Job drawing, mm, ordinate dimensions from the low corner. One solid piece. Round coordinates to 2 decimals unless told otherwise and drop trailing zeros. Order: outer loops, then holes, each group sorted by start corner. A loop starts at its lowest first (then second) coordinate and runs counter-clockwise, first axis right, second up. Notation, with made-up numbers: (-30, 5) -> (12, 5) arc R21 cw to (12, 27) -> close; hole circle Ø6 at (87, 13). An arc over 180 degrees is marked (long way). Use CSV: the item, a comma, the result in double quotes.
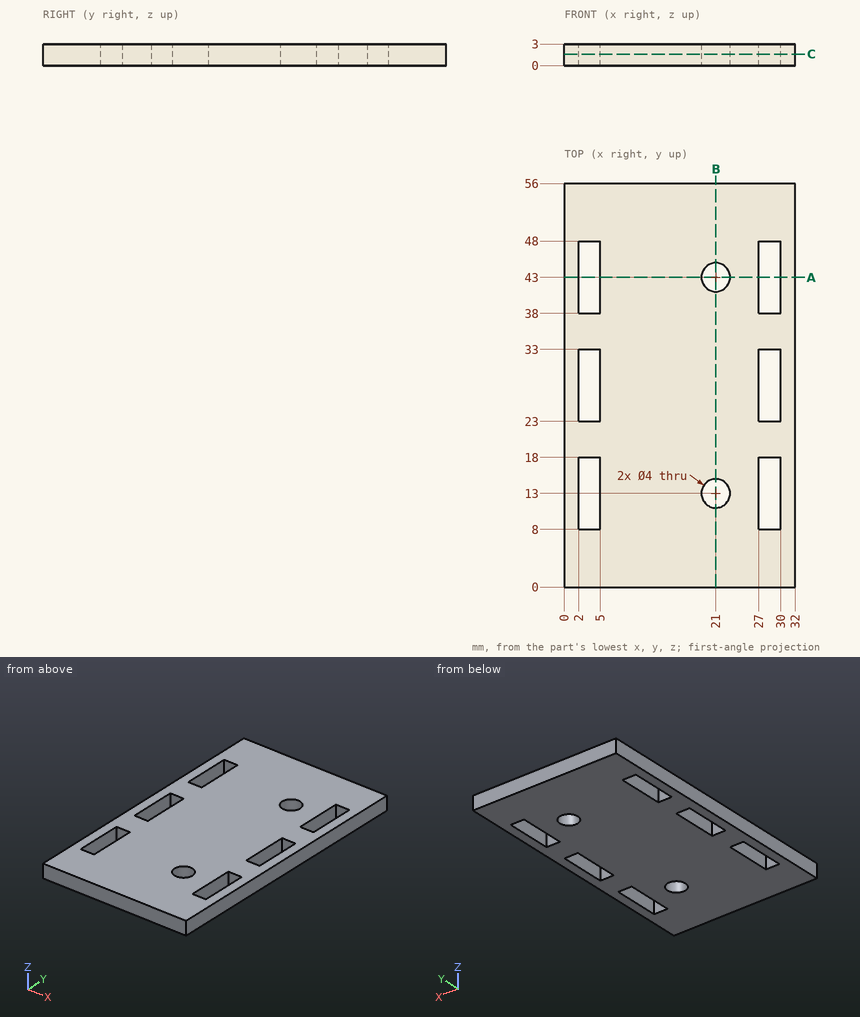
(1) Cut at A-A, the plane y = 43. Give the cut face in (x, z).
Reply:
outline,"(0, 0) -> (2, 0) -> (2, 3) -> (0, 3) -> close; (5, 0) -> (19, 0) -> (19, 3) -> (5, 3) -> close; (23, 0) -> (27, 0) -> (27, 3) -> (23, 3) -> close; (30, 0) -> (32, 0) -> (32, 3) -> (30, 3) -> close"
(2) Drop a flat-ended pin along its axis: P1, Ø3, axis at x = 21, y = 13, coming from the -Z side. Give the stop position or say it passes through.
Reply:
P1,"through"
(3) Cut at B-B, the plane x = 21. Give the cut face in (y, z).
Reply:
outline,"(0, 0) -> (11, 0) -> (11, 3) -> (0, 3) -> close; (15, 0) -> (41, 0) -> (41, 3) -> (15, 3) -> close; (45, 0) -> (56, 0) -> (56, 3) -> (45, 3) -> close"
(4) Cut at C-C, the plane z = 1.6. State how many separate pieces and enclosed holes the cut face has, then the cut area to 3 significant figures.
Reply:
separate pieces,"1"
enclosed holes,"8"
area,"1,590 mm2"
(5) Probe probe 1 along Y at (x, z) = (21, 1.05); probe 2 along X at (y, z) = (25.5, 0.2); probe 3 along X at (y, z) = (12.5, 1). List the from-to ranges inside material, lowest first. Write a range as [from, to].
Reply:
probe 1,"[0, 11], [15, 41], [45, 56]"
probe 2,"[0, 2], [5, 27], [30, 32]"
probe 3,"[0, 2], [5, 19.06], [22.94, 27], [30, 32]"
